Model file for the job. Use its own axes, mm. Face numbers are marked on the shaded views. A direction names the side the tool comes from. Give positions to 0.01 mm unless a question says otherwise; leave off trailing zeros. Order: outer loops, then holes, each group sorted by start corner. A loop starts at its lowest first (then second) coordinate and runs counter-clockwise, first axis right, second up. Notation, with made-up numbers: (32.5, 21) - (57.5, 21) arc R26 ccw to (57.5, 46) - close; hole circle Ø2 at (-22, 46.5). An arc over 180 degrees is marked (long way). Use CSV: the item, a comma, the result in double quotes. Start each with the question number.
(1) Pull direction Z, two halves, no side cores. Call the marked faces 1, 2, 3 and 4: +Z half, -Z half, draft (parallel to the pull), parting line (faces both ways), or undercut.
(2) Band-saw the part on B-B, the plane y = 41.5. Give the cut face in (x, z).
(3) Probe L1, parallel to X at y = 24.5, z = 0; L2, parallel to Z at x = -1.5, y = 21.5; L3, parallel to Z at x = -10.5, y = 26. List the from-to ranges inside material, lowest first.
(4) Drop flat-ended pins along their axis: pin 1 Ø10 at (y, z) = (26.5, 37) entering from -X; pin 2 Ø1.1 at (x, y) = (-1.5, 22.5) entering from -Z; pin 3 Ø1 at (x, y) = (-9.5, 22.5) entering from +Z; pin 4 Ø3 at (x, z) = (39.5, -5) entering from -Y. Give the stop position or say it passes through.
(5) Band-saw the part on A-A, the plane y = 12. Give the cut face in (x, z).
(6) Tool access for the marked faces 5 and 6: list every direction of +Z, -Z, +X, -X, +Y, -Y with a clear straight run to the whole face (end or side of a thin tool).
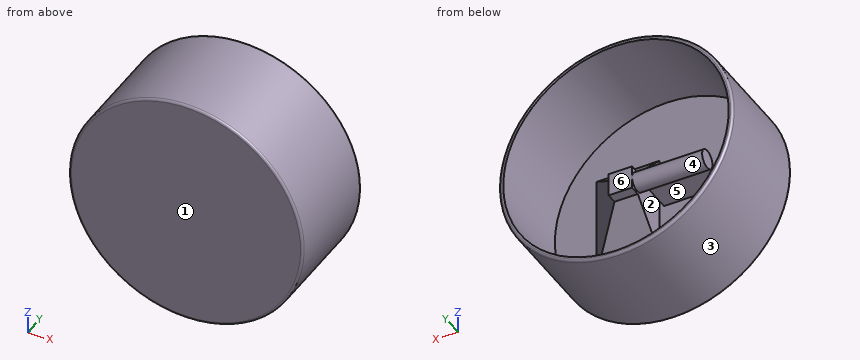
from build123d import *

# Parameters (mm, degrees)
SKETCH1_R                = 50.05
BOSS_EXTRUDE1_DEPTH      = 45
SKETCH3_R                = 48.25
CUT_EXTRUDE2_DEPTH       = 40
SKETCH4_W                = 10
SKETCH4_H                = 10
BOSS_EXTRUDE2_DEPTH      = 21.5
SKETCH5_R                = 4
BOSS_EXTRUDE3_DEPTH      = 30
BOSS_EXTRUDE4_REACH      = 83.302
BOSS_EXTRUDE4_END_RADIUS = 4
SKETCH6_W                = 28.184708005
SKETCH6_H                = 0.2
FILLET1_R                = 1
CHAMFER1_SIZE            = 17
SKETCH7_W                = 4.566458064
SKETCH7_H                = 1.143701811
SKETCH7_W_2              = 4.660128999
SKETCH7_H_2              = 1.247674702
SKETCH7_W_3              = 3.257159631
SKETCH7_H_3              = 1.039728918
SKETCH7_W_4              = 2.28740362
SKETCH7_H_4              = 1.66356627
SKETCH7_W_5              = 2.391376512
SKETCH7_H_5              = 1.975484945
SKETCH7_W_6              = 1.695413964
SKETCH7_H_6              = 1.039728919
SKETCH7_W_7              = 1.401040737
SKETCH7_H_7              = 0.457148196
CUT_EXTRUDE3_DEPTH       = 0.2


with BuildPart() as part:
    # Sketch1 → Boss-Extrude1 (new body)
    with BuildSketch(Plane(origin=(0, 0, 0), x_dir=(1, 0, 0), z_dir=(0, 1, 0))):
        with Locations(Location((0, 0, 0), (0, 0, 90))):
            Circle(SKETCH1_R)
    extrude(amount=BOSS_EXTRUDE1_DEPTH)

    # Sketch3 → Cut-Extrude2 (cut)
    with BuildSketch(Plane(origin=(0, 45, 0), x_dir=(1, 0, 0), z_dir=(0, 1, 0))):
        with Locations(Location((0, 0, 0), (0, 0, 270))):
            Circle(SKETCH3_R)
    extrude(amount=-CUT_EXTRUDE2_DEPTH, mode=Mode.SUBTRACT)

    # Sketch4 → Boss-Extrude2 (add)
    with BuildSketch(Plane(origin=(0, 5, 0), x_dir=(1, 0, 0), z_dir=(0, 1, 0))):
        with Locations((8.34608558, 0)):
            Rectangle(SKETCH4_W, SKETCH4_H)
    extrude(amount=BOSS_EXTRUDE2_DEPTH)

    # Sketch5 → Boss-Extrude3 (add)
    with BuildSketch(Plane.ZY.offset(-3.34608558)):
        with Locations(Location((0, 22.5, 0), (0, 0, 90))):
            Circle(SKETCH5_R)
    extrude(amount=BOSS_EXTRUDE3_DEPTH)

    # Boss-Extrude4: up to this cylinder (the profile starts outside it)
    boss_extrude4_end = Plane(origin=(-12.56156, 22.5, 0), z_dir=(1, 0, 0)) * Cylinder(BOSS_EXTRUDE4_END_RADIUS, 175.604, mode=Mode.PRIVATE)
    # Sketch6 → Boss-Extrude4 (add, up to the surface)
    with BuildSketch(Plane(origin=(0, 5, 0), x_dir=(1, 0, 0), z_dir=(0, 1, 0)), mode=Mode.PRIVATE) as boss_extrude4_sk1:
        with Locations((-12.561560418, -0.1)):
            Rectangle(SKETCH6_W, SKETCH6_H)
    boss_extrude4_tool1 = extrude(boss_extrude4_sk1.sketch, amount=BOSS_EXTRUDE4_REACH, mode=Mode.PRIVATE) - boss_extrude4_end
    add(boss_extrude4_tool1.solids().sort_by_distance((-12.56156, 5, 0.1))[0])

    # Fillet1
    fillet1_edges = [part.edges().sort_by_distance(p)[0] for p in [
        (0, 0, 50.05),
        (0, 45, 50.05),
    ]]
    fillet(fillet1_edges, radius=FILLET1_R)

    # Chamfer1
    chamfer1_edges = [part.edges().sort_by_distance(p)[0] for p in [
        (8.34608558, 5, 5),
        (13.34608558, 5, 0),
        (8.34608558, 5, -5),
    ]]
    chamfer(chamfer1_edges, length=CHAMFER1_SIZE)

    # Sketch7 → Cut-Extrude3 (cut)
    with BuildSketch(Plane.XY):
        with Locations((-20.640838481, 22.591171411)):
            Rectangle(SKETCH7_W, SKETCH7_H)
        with Locations((-10.266782469, 22.539184965)):
            Rectangle(SKETCH7_W_2, SKETCH7_H_2)
        with Locations((-2.115257482, 22.435212073)):
            Rectangle(SKETCH7_W_3, SKETCH7_H_3)
        with Locations((7.901126588, 17.340540373)):
            Rectangle(SKETCH7_W_4, SKETCH7_H_4)
        with Locations((13.775594976, 17.184581036)):
            Rectangle(SKETCH7_W_5, SKETCH7_H_5)
        with Locations((3.589327362, 22.345655797)):
            Rectangle(SKETCH7_W_6, SKETCH7_H_6)
        with Locations((6.850941154, 20.421535498)):
            Rectangle(SKETCH7_W_7, SKETCH7_H_7)
    extrude(amount=-CUT_EXTRUDE3_DEPTH, mode=Mode.SUBTRACT)


solid = part.part
Answer block:
1,face 1,"draft"
1,face 2,"undercut"
1,face 3,"parting line"
1,face 4,"undercut"
2,outline,"circle Ø100.1 at (0, 0); hole circle Ø96.5 at (0, 0)"
3,L1,"x = -50.05 to -48.25, -26.65 to 13.35, 48.25 to 50.05"
3,L2,"z = -50.03 to -48.23, -3.87 to 3.87, 48.23 to 50.03"
3,L3,"z = -48.94 to -47.09, -1.94 to 1.94, 47.09 to 48.94"
4,pin 1,"stops at x = -38.48"
4,pin 2,"stops at z = -50.04"
4,pin 3,"stops at z = 49.23"
4,pin 4,"stops at y = 0"
5,outline,"circle Ø100.1 at (0, 0); (-26.65, 0) - (1.53, 0) - (1.53, 0.2) - (-26.65, 0.2) - close; (3.35, -15) - (23.35, -15) - (23.35, 15) - (3.35, 15) - close; hole circle Ø96.5 at (0, 0)"
6,face 5,"none"
6,face 6,"+Y"
